```python
from build123d import *

# Parameters (mm, degrees)
F0_R      = 50
F1_DEPTH  = 4
F3_DEPTH  = 5.8
F4_DEPTH  = 5.8
F5_DEPTH  = 5.8
F6_R      = 45
F7_DEPTH  = 4
F8_W      = 6
F8_H      = 6
F9_DEPTH  = 4
F10_R     = 22.5
F11_DEPTH = 25
F12_W     = 47.8333383799
F12_H     = 64.1666669399
F13_DEPTH = 45
F14_SIZE  = 15
F15_SIZE  = 5
F16_R     = 5
F18_DEPTH = 43
F19_R     = 10


with BuildPart() as f1:
    # F0 (on Top) → F1 (new body)
    with BuildSketch(Plane.XY):
        Circle(F0_R)
    extrude(amount=F1_DEPTH)

    # F2 (on face) → F3 (join)
    with BuildSketch(Plane.XY.offset(4)):
        with BuildLine():
            ThreePointArc((5, 49.7493718553), (2.503138753, 49.9373036555), (0, 50))
            ThreePointArc((0, 50), (-2.503138753, 49.9373036555), (-5, 49.7493718553))
            Line((-5, 49.7493718553), (-5, 44.5003296036))
            Line((-5, 44.5003296036), (5, 44.5003296036))
            Line((5, 44.5003296036), (5, 49.7493718553))
        make_face()
    extrude(amount=F3_DEPTH)

    # F2 (on face) → F4 (join)
    with BuildSketch(Plane.XY.offset(4)):
        with BuildLine():
            ThreePointArc((0, -50), (2.503138753, -49.9373036555), (5, -49.7493718553))
            Line((5, -49.7493718553), (5, -44))
            Line((5, -44), (-5, -44))
            Line((-5, -44), (-5, -49.7493718553))
            ThreePointArc((-5, -49.7493718553), (-2.503138753, -49.9373036555), (0, -50))
        make_face()
    extrude(amount=F4_DEPTH)

    # F2 (on face) → F5 (join)
    with BuildSketch(Plane.XY.offset(4)):
        with BuildLine():
            Line((-44, 5), (-49.7493718553, 5))
            ThreePointArc((-49.7493718553, 5), (-49.9373036555, 2.503138753), (-50, 0))
            ThreePointArc((-50, 0), (-49.9373036555, -2.503138753), (-49.7493718553, -5))
            Line((-49.7493718553, -5), (-44, -5))
            Line((-44, -5), (-44, 5))
        make_face()
        with BuildLine():
            ThreePointArc((50, 0), (49.9373036555, 2.503138753), (49.7493718553, 5))
            Line((49.7493718553, 5), (44, 5))
            Line((44, 5), (44, -5))
            Line((44, -5), (49.7493718553, -5))
            ThreePointArc((49.7493718553, -5), (49.9373036555, -2.503138753), (50, 0))
        make_face()
    extrude(amount=F5_DEPTH)

    # F6 (on Top) → F7 (cut)
    with BuildSketch(Plane.XY):
        Circle(F6_R)
    extrude(amount=F7_DEPTH, mode=Mode.SUBTRACT)

    # F8 (on Top) → F9 (join)
    with BuildSketch(Plane.XY):
        Polygon((6, 46.8811020255), (-6, 46.8811020255), (-6, 6), (0, 6), (6, 6), align=None)
        with Locations((-3, 3)):
            Rectangle(F8_W, F8_H)
        Polygon((-6, 0), (-6, 6), (-46.5700030327, 6), (-46.5700030327, -6), (-6, -6), align=None)
        Polygon((46.8255914748, 6), (6, 6), (6, 0), (6, -6), (46.8255914748, -6), align=None)
        with Locations((3, 3)):
            Rectangle(F8_W, F8_H)
        with Locations((-3, -3)):
            Rectangle(F8_W, F8_H)
        with Locations((3, -3)):
            Rectangle(F8_W, F8_H)
        Polygon((0, -6), (-6, -6), (-6, -46.7753745615), (6, -46.7753745615), (6, -6), align=None)
    extrude(amount=F9_DEPTH)

    # F10 (on face) → F11 (cut)
    with BuildSketch(Plane(origin=(0, 0, 0), x_dir=(1, 0, 0), z_dir=(0, 0, -1))):
        Circle(F10_R)
    extrude(amount=-F11_DEPTH, mode=Mode.SUBTRACT)

    # F12 (on Top) → F13 (join)
    with BuildSketch(Plane.XY):
        with Locations((-0.1458320767, -0.7291669026)):
            Rectangle(F12_W, F12_H)
    extrude(amount=F13_DEPTH)

    # F14
    f14_edges = [f1.edges().sort_by_distance(p)[0] for p in [
        (-24.062501, 31.354167, 22.5),
        (23.770837, 31.354167, 22.5),
        (23.770837, -32.8125, 22.5),
        (-24.062501, -32.8125, 22.5),
    ]]
    chamfer(f14_edges, length=F14_SIZE)

    # F15
    f15_edges = [f1.edges().sort_by_distance(p)[0] for p in [
        (-9.062501, 31.354167, 22.5),
        (8.770837, 31.354167, 22.5),
        (-24.062501, -17.8125, 22.5),
        (-9.062501, -32.8125, 22.5),
        (8.770837, -32.8125, 22.5),
        (23.770837, -17.8125, 22.5),
        (23.770837, 16.354167, 22.5),
        (-24.062501, 16.354167, 22.5),
    ]]
    chamfer(f15_edges, length=F15_SIZE)

    # F16
    f16_edges = [f1.edges().sort_by_distance(p)[0] for p in [
        (-24.062501, 11.354167, 22.5),
        (-20.526967, 19.8897, 22.5),
        (-12.598035, 27.818633, 22.5),
        (-4.062501, 31.354167, 24.5),
        (3.770837, 31.354167, 24.5),
        (12.306371, 27.818633, 22.5),
        (20.235303, 19.8897, 22.5),
        (23.770837, 11.354167, 22.5),
        (23.770837, -12.8125, 22.5),
        (20.235303, -21.348034, 22.5),
        (12.306371, -29.276966, 22.5),
        (3.770837, -32.8125, 24.5),
        (-4.062501, -32.8125, 24.5),
        (-24.062501, -12.8125, 22.5),
        (-20.526967, -21.348034, 22.5),
        (-12.598035, -29.276966, 22.5),
    ]]
    fillet(f16_edges, radius=F16_R)

    # F17 (on face) → F18 (cut)
    with BuildSketch(Plane(origin=(0, 0, 0), x_dir=(1, 0, 0), z_dir=(0, 0, -1))):
        with BuildLine():
            Line((11.3142130134, 19.4022327268), (11.1320833255, 19.7139199305))
            ThreePointArc((11.1320833255, 19.7139199305), (0, 26), (-11.1320833255, 19.7139199305))
            ThreePointArc((-11.1320833255, 19.7139199305), (-11.9963062924, 7.9911443085), (-3.0526367469, 0.3634890539))
            ThreePointArc((-3.0526367469, 0.3634890539), (0, 0.7269781077), (3.0526367469, 0.3634890539))
            ThreePointArc((3.0526367469, 0.3634890539), (10.2147999909, 4.9589887983), (13, 13))
            ThreePointArc((13, 13), (12.5714909453, 16.3102289065), (11.3142130134, 19.4022327268))
        make_face()
        with BuildLine():
            ThreePointArc((11.3142130134, 19.4022327268), (11.2242301322, 19.5587085572), (11.1320833255, 19.7139199305))
            Line((11.1320833255, 19.7139199305), (11.3142130134, 19.4022327268))
        make_face()
        with BuildLine():
            ThreePointArc((-3.0526367469, 0.3634890539), (-11.9963062924, 7.9911443085), (-11.1320833255, 19.7139199305))
            Line((-11.1320833255, 19.7139199305), (-20.499, 4.1830083316))
            Line((-20.499, 4.1830083316), (-20.499, -4.1830083316))
            Line((-20.499, -4.1830083316), (-10.9868011053, -19.2221370497))
            ThreePointArc((-10.9868011053, -19.2221370497), (-12.0488854783, -7.3920016371), (-3.0526367469, 0.3634890539))
        make_face()
        with BuildLine():
            Line((20.2073358467, 4.1830083316), (11.3142130134, 19.4022327268))
            ThreePointArc((11.3142130134, 19.4022327268), (12.5714909453, 16.3102289065), (13, 13))
            ThreePointArc((13, 13), (10.2147999909, 4.9589887983), (3.0526367469, 0.3634890539))
            ThreePointArc((3.0526367469, 0.3634890539), (10.2147999909, -4.2320106906), (13, -12.2730218923))
            ThreePointArc((13, -12.2730218923), (12.5358890301, -15.7156206526), (11.1766944269, -18.9124120515))
            Line((11.1766944269, -18.9124120515), (20.2073358467, -4.1830083316))
            Line((20.2073358467, -4.1830083316), (20.2073358467, 4.1830083316))
        make_face()
        with BuildLine():
            ThreePointArc((3.0526367469, 0.3634890539), (0, 0), (-3.0526367469, 0.3634890539))
            ThreePointArc((-3.0526367469, 0.3634890539), (-12.0488854783, -7.3920016371), (-10.9868011053, -19.2221370497))
            ThreePointArc((-10.9868011053, -19.2221370497), (0, -25.2730218923), (10.9868011053, -19.2221370497))
            Line((10.9868011053, -19.2221370497), (11.1766944269, -18.9124120515))
            ThreePointArc((11.1766944269, -18.9124120515), (12.5358890301, -15.7156206526), (13, -12.2730218923))
            ThreePointArc((13, -12.2730218923), (10.2147999909, -4.2320106906), (3.0526367469, 0.3634890539))
        make_face()
        with BuildLine():
            Line((11.1766944269, -18.9124120515), (10.9868011053, -19.2221370497))
            ThreePointArc((10.9868011053, -19.2221370497), (11.0828297806, -19.0679379369), (11.1766944269, -18.9124120515))
        make_face()
        with BuildLine():
            ThreePointArc((3.0526367469, 0.3634890539), (0, 0.7269781077), (-3.0526367469, 0.3634890539))
            ThreePointArc((-3.0526367469, 0.3634890539), (0, 0), (3.0526367469, 0.3634890539))
        make_face()
    extrude(amount=-F18_DEPTH, mode=Mode.SUBTRACT)

    # F19
    f19_edges = [f1.edges().sort_by_distance(p)[0] for p in [
        (-20.499, 4.183008, 21.5),
        (20.207336, 4.183008, 21.5),
        (-20.499, -4.183008, 21.5),
        (20.207336, -4.183008, 21.5),
    ]]
    fillet(f19_edges, radius=F19_R)


solid = f1.part
```
Design review of the part built by this model. Coordinates are the model's own, in mm. A direction names the side the tool comes from. Coordinates: 2 decimals unless noted, no trailing zeros. Write each loop counter-clockwise with the first axis right and the second up, starting at its lowest first coordinate (ties: lowest second). Pieces come first, ordered by that corner, then holes.
1) To check wall thickness, follow L1, parallel to X at y = -7.5, z = 3.5; L2, parallel to Z at x = 6, y = 15.5; L3, parallel to Z at x = -24, y = 43. State the ranges of each line that lie inside material, in increasing order.
2) Mouldability with a two-part tool opening along X and no side actions: class faces 6 (the flat face through (0, 31.354, 24)), 7 (the flat face through (0, -1, 43)), 8 (the flat face through (5, -47, 7)) as +X half, -X half, draft (parallel to the pull), parting line (faces both ways), or undercut.
3) Add section A-A (z = 8.5). State how many separate pieces and enclosed holes the cut face has, plus the area to 3 significant figures.
4) Insertion check: pin 1 (1.7 mm diameter, centred on y = -47, z = 6.5, fed in from -X); pin 2 (11 mm diameter, centred on y = -4.5, z = 31.5, fed in from +X); pin 3 (11 mm diameter, centred on y = -5.5, z = 28, fed in from -X). Each pin has a flat end and moves straight along its axis. Give the tip position at first contact, or say it passes through.
5) Machinability: for faces 1 (the flat face through (-15.042, -13.232, 21.199)), 2 (the flat face through (-5, 47, 7)), 3 (the flat face through (5, 47, 7)), 4 (the flat face through (6, -38, 2)), 5 (the flat face through (0, 0, 45)), which of the approach directions +Z, -Z, +X, -X, +Y, -Y give a long, thin tool a straight path to every point of the face, cutting with its end or side? Answer none if there is none.
6) Add section B-B (x = 32.5). Write out the cut boundary in (y, z).
Check result:
1. L1: x = -49.43 to -44.37, -24.06 to -18.5, 18.27 to 23.77, 44.37 to 49.43
1. L2: z = 43 to 45
1. L3: z = 0 to 4
2. face 6: draft
2. face 7: undercut
2. face 8: +X half
3. separate pieces: 5
3. enclosed holes: 1
3. area: 1,290 mm2
4. pin 1: stops at x = -5
4. pin 2: stops at x = 23.77
4. pin 3: stops at x = -24.06
5. face 1: -Z
5. face 2: +Z, -X, +Y
5. face 3: +Z, +X, +Y
5. face 4: +Z, -Z
5. face 5: +Z, +X, -X, +Y, -Y
6. outline: (-38, 0) - (-31.12, 0) - (-31.12, 4) - (-38, 4) - close; (-6, 0) - (6, 0) - (6, 4) - (-6, 4) - close; (31.12, 0) - (38, 0) - (38, 4) - (31.12, 4) - close
